```python
from build123d import *

# Parameters (mm, degrees)
F1_DEPTH = 11.43
F2_W     = 81.271418
F2_H     = 115.942701
F3_DEPTH = 0.1778
F4_W     = 86.214885
F4_H     = 150.880255
F5_DEPTH = 0.0254
F6_R     = 3.101618
F7_DEPTH = 3.81
F8_R     = 2.925267
F9_DEPTH = 0.0254


with BuildPart() as f1:
    # F0 (on Top) → F1 (new body)
    with BuildSketch(Plane.XY):
        Polygon((47.590654, 76.434568), (0, 76.434568), (-41.661378, 76.434568), (-41.661378, 0), (-41.661378, -76.72172), (-41.661378, -77.591054), (0, -77.591054), (47.590654, -77.591054), align=None)
    extrude(amount=F1_DEPTH)

    # F2 (on face) → F3 (cut)
    with BuildSketch(Plane.XY.offset(11.43)):
        with Locations((3.015559, -0.350732)):
            Rectangle(F2_W, F2_H)
    extrude(amount=-F3_DEPTH, mode=Mode.SUBTRACT)

    # F4 (on face) → F5 (cut)
    with BuildSketch(Plane.XY.offset(11.43)):
        with Locations((3.301713, -0.995736)):
            Rectangle(F4_W, F4_H)
    extrude(amount=-F5_DEPTH, mode=Mode.SUBTRACT)

    # F6 (on face) → F7 (cut)
    with BuildSketch(Plane.XY.offset(11.4046)):
        with Locations((-30.738983, 62.852658)):
            Circle(F6_R)
    extrude(amount=-F7_DEPTH, mode=Mode.SUBTRACT)

    # F8 (on face) → F9 (join)
    with BuildSketch(Plane.XY.offset(7.5946)):
        with Locations((-30.738983, 62.852658)):
            Circle(F8_R)
    extrude(amount=F9_DEPTH)


solid = f1.part
```
For this review, take the finished solid that the model builds, in its own axes (mm). A direction names the side the tool comes from. Coordinates: 2 decimals unless noted, no trailing zeros. Answer as CSV lines item,"result".
Q1. Clearance check with flat-ended pins moving along their axes: pin 1 Ø12 at (x, y) = (20.5, -43) entering from +Z; pin 2 Ø1.9 at (x, y) = (-31.5, 61.5) entering from +Z; pin 3 Ø6.5 at (x, y) = (-30, 64) entering from +Z. State where each tip first meets the part, or that it passes through.
Model answer:
pin 1,"stops at z = 11.25"
pin 2,"stops at z = 7.62"
pin 3,"stops at z = 11.4"
Q2. For faces 5 (the face through (2, 0, 11.252)), 6 (the face through (2, -77.591, 6)), list the 3-axis set-ups (+Z, -Z, +X, -X, +Y, -Y) from which the entire face can be reached by the end or side of a thin tool; tool diameter is ignored.
Model answer:
face 5,"+Z"
face 6,"+Z, -Z, +X, -X, -Y"
Q3. Draft analysis for pull direction Y (two halves, no side actions). For faces 1 (the face through (-31, 63, 7.62)), 2 (the face through (-31.411, 59.825, 9.526)), 3 (the face through (47.591, -2, 6)), 4 (the face through (4, 76.435, 6)), state which applies: released by +Y, released by -Y, zero draft, split by the parting line, or undercut.
Model answer:
face 1,"undercut"
face 2,"undercut"
face 3,"zero draft"
face 4,"released by +Y"
Q4. Wall thickness on line 1 along Z through (x, y) = (-3, -15.5): over which ranges is the line inside the solid? List them lowest first. Write a range as [from, to].
Model answer:
line 1,"z = [0, 11.25]"
